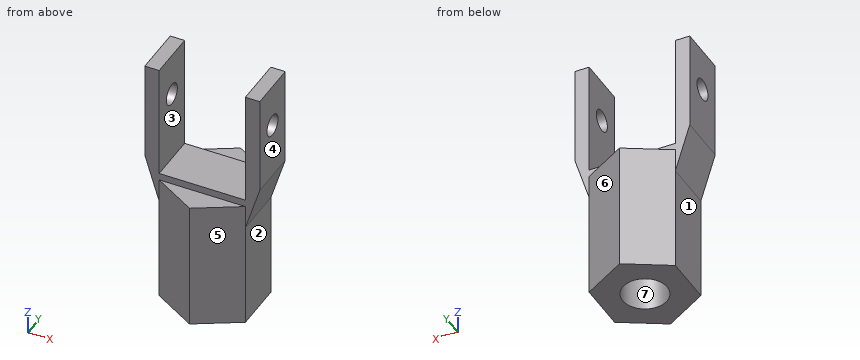
Autodesk Inventor part; units mm, degrees
ref_plane "YZ Plane" through (0, 0, 0) normal (1, 0, 0) x (0, 1, 0)
ref_plane "XZ Plane" through (0, 0, 0) normal (0, 1, 0) x (-1, 0, 0)
ref_plane "XY Plane" through (0, 0, 0) normal (0, 0, 1) x (1, 0, 0)
sketch "Sketch1" plane through (0, 0, 0) normal (0, 0, 1) x (1, 0, 0)
  line L0 (8, 0.0718) -> (2, 3.5359)
  line L1 (2, 3.5359) -> (2, 10.4641)
  line L2 (2, 10.4641) -> (8, 13.9282)
  line L3 (8, 13.9282) -> (14, 10.4641)
  line L4 (14, 10.4641) -> (14, 3.5359)
  line L5 (14, 3.5359) -> (8, 0.0718)
  point P0 (0, 0)
  point P1 (8, 7)
  dimension "d1" = 12
extrude "Extrusion1" add sketch "Sketch1" along normal blind 18
sketch "Sketch2" plane through (0, 0, 0) normal (0, 0, -1) x (-1, 0, 0)
  circle A0 centre (-8, 7) radius 3.1
  point P0 (0, 0)
  dimension "d5" = 6.2
extrude "Extrusion2" cut sketch "Sketch2" against normal blind 14
sketch "Sketch3" plane through (0, 0, 18) normal (0, 0, 1) x (1, 0, 0)
  line L0 (14, 3.5359) -> (8, 0.0718)
  line L1 (14, 3.5359) -> (2, 3.5359)
  line L2 (2, 3.5359) -> (2, 10.4641)
  line L3 (2, 10.4641) -> (14, 10.4641)
  line L4 (14, 10.4641) -> (14, 3.5359)
  point P0 (0, 0)
  dimension "d12" = 6.9282
extrude "Extrusion3" add sketch "Sketch3" along normal blind 17
sketch "Sketch4" plane through (2, 10.4641, 18) normal (0, 1, 0) x (1, 0, 0)
  line L0 (12, 0) -> (12, -17)
  line L1 (12, -17) -> (14, -17)
  line L2 (0, 0) -> (0, -17)
  line L3 (12, 0) -> (12, -17)
  line L4 (0, -17) -> (-2, -17)
  line L5 (0, 0) -> (0, -17)
  line L6 (14, -17) -> (14, -3.1957)
  line L7 (-2, -3.1957) -> (0, 3.2792)
  line L8 (14, -3.1957) -> (12, 3.2792)
  line L9 (12, 18) -> (12, 0)
  line L10 (0, 0) -> (0, 3.2792)
  line L11 (12, 0) -> (12, 3)
  line L12 (-2, -17) -> (-2, -3.1957)
  point P0 (-2, 18)
  dimension "d10" = 2
  dimension "d11" = 2
extrude "Extrusion4" add sketch "Sketch4" against normal blind 6.9282
sketch "Sketch5" plane through (2, 10.4641, 18) normal (0, 1, 0) x (1, 0, 0)
  line L0 (14, -17) -> (14, -17)
  line L1 (0, -17) -> (12, -17)
  line L2 (12, -17) -> (12, -1)
  line L3 (12, -1) -> (0, -1)
  line L4 (0, -1) -> (0, -17)
  point P0 (-2, 18)
  point P1 (-2, -17)
extrude "Extrusion5" cut sketch "Sketch5" against normal through all
sketch "Sketch6" plane through (0, 10.4641, 21.1957) normal (-1, 0, 0) x (0, 0, 1)
  line L0 (13.8043, 0) -> (13.8043, -6.9282)
  circle A0 centre (7.8043, -3.4641) radius 1.5
  point P0 (-21.1957, -10.4641)
  dimension "d18" = 3
extrude "Extrusion6" cut sketch "Sketch6" against normal through all
properties part number "supportrod"
Geometry check sheet. Reference: the model listing, model coordinates, mm. Face numbers are marked on the shaded views. A direction names the side the tool comes from. Give positions to 0.01 mm unless a question says otherwise; leave off trailing zeros. Loops run counter-clockwise (first coordinate to the right, second up) from the corner with the lowest first, then second, coordinate; pieces in that order, holes last. Notation, with made-up numbers: M 74.5,-13.5 L 93.5,-13.5 A27 cw 93.5,7.5 Z; hole C 27.25,-30 d2. An arc over 180 degrees is marked long. Write item = value, one per line. Start each with the question number.
1. Section check C-C, the plane z = 12.5. Enter the section's corners in (x, y).
2. Section check D-D, the plane y = 9.25. Enter the section's corners in (x, z).
3. Go/stop test with flat-tipped pins: P1, Ø8, axis at y = 7.5, z = 4.5, coming from the +X side; P2, Ø3, axis at x = 7, y = 10, coming from the +Z side; P3, Ø1, axis at x = 8, y = 2, coming from the +Z side. Record where each tip stops, or that it passes through.
4. Tool access check on the marked faces 1, 2 and 3. Record the directions out of +Z, -Z, +X, -X, +Y, -Y that give a thin tool (end or side, any length) a straight path to the whole face; none if there is none.
5. Draft check along Y on the marked faces 4, 5, 6 and 7. Enter one of: +Y half, -Y half, draft (parallel to the pull), parting line (faces both ways), or undercut.
6. Section check B-B, the plane y = 7. Enter the section's corners in (x, z).
7. Thickness scan on probe 1 along X at (y, z) = (6.25, 31.5); probe 2 along Y at (x, z) = (0.6, 29); probe 3 along Z at (x, y) = (5.5, 6). Record the ranges inside material, lowest first.
8. Section check A-A, the plane z = 31.5. Enter the section's corners in (x, y).
Values follow:
q1.outline = M 2,3.54 L 8,0.07 L 14,3.54 L 14,10.46 L 8,13.93 L 2,10.46 Z; hole C 8,7 d6.2
q2.outline = M 0,21.2 L 2,14.72 L 2,0 L 5.87,0 L 5.87,14 L 10.13,14 L 10.13,0 L 14,0 L 14,14.72 L 16,21.2 L 16,35 L 14,35 L 14,19 L 2,19 L 2,35 L 0,35 Z
q3.P1 = 14
q3.P2 = 19
q3.P3 = 18
q4.face_1 = -Z, -X, +Y, -Y
q4.face_2 = -Z, +X, +Y, -Y
q4.face_3 = +Z, +Y, -Y
q5.face_4 = draft
q5.face_5 = -Y half
q5.face_6 = +Y half
q5.face_7 = undercut
q6.outline = M 0,21.2 L 2,14.72 L 2,0 L 4.9,0 L 4.9,14 L 11.1,14 L 11.1,0 L 14,0 L 14,14.72 L 16,21.2 L 16,27.5 L 14,27.5 L 14,19 L 2,19 L 2,27.5 L 0,27.5 Z; M 0,30.5 L 2,30.5 L 2,35 L 0,35 Z; M 14,30.5 L 16,30.5 L 16,35 L 14,35 Z
q7.probe_1 = 0 to 2, 14 to 16
q7.probe_2 = 3.54 to 5.5, 8.5 to 10.46
q7.probe_3 = 14 to 19
q8.outline = M 0,3.54 L 2,3.54 L 2,10.46 L 0,10.46 Z; M 14,3.54 L 16,3.54 L 16,10.46 L 14,10.46 Z
